from build123d import *

# Parameters (mm, degrees)
SKETCH_1_R      = 1.5
EXTRUDE_1_DEPTH = 3


with BuildPart() as part:
    # 스케치1 → 보스-돌출1 (new body)
    with BuildSketch(Plane.XY):
        Polygon((-47.224852071, 90.964497041), (191.775147929, 90.964497041), (191.775147929, -71.035502959), (-158.224852071, -71.035502959), (-158.224852071, 90.964497041), (-158.224852071, 112.964497041), (-47.224852071, 112.964497041), align=None)
        with Locations((-108.224852071, 78.964497041)):
            Circle(SKETCH_1_R, mode=Mode.SUBTRACT)
        with Locations((-68.224852071, 78.964497041)):
            Circle(SKETCH_1_R, mode=Mode.SUBTRACT)
        with Locations((101.775147929, 78.964497041)):
            Circle(SKETCH_1_R, mode=Mode.SUBTRACT)
        with Locations((141.775147929, 78.964497041)):
            Circle(SKETCH_1_R, mode=Mode.SUBTRACT)
        with Locations((141.775147929, -41.035502959)):
            Circle(SKETCH_1_R, mode=Mode.SUBTRACT)
        with Locations((41.775147929, -41.035502959)):
            Circle(SKETCH_1_R, mode=Mode.SUBTRACT)
        with Locations((-8.224852071, -41.035502959)):
            Circle(SKETCH_1_R, mode=Mode.SUBTRACT)
        with Locations((-108.224852071, -41.035502959)):
            Circle(SKETCH_1_R, mode=Mode.SUBTRACT)
        with Locations((-152.024852071, 110.064497041)):
            Circle(SKETCH_1_R, mode=Mode.SUBTRACT)
        with Locations((-50.424852071, 110.064497041)):
            Circle(SKETCH_1_R, mode=Mode.SUBTRACT)
        with Locations((-41.224852071, 86.464497041)):
            Circle(SKETCH_1_R, mode=Mode.SUBTRACT)
        with Locations((185.775147929, 86.464497041)):
            Circle(SKETCH_1_R, mode=Mode.SUBTRACT)
        with Locations((185.775147929, -64.535502959)):
            Circle(SKETCH_1_R, mode=Mode.SUBTRACT)
        with Locations((-41.224852071, -64.535502959)):
            Circle(SKETCH_1_R, mode=Mode.SUBTRACT)
        with Locations((-50.424852071, -64.535502959)):
            Circle(SKETCH_1_R, mode=Mode.SUBTRACT)
        with Locations((-152.024852071, -64.535502959)):
            Circle(SKETCH_1_R, mode=Mode.SUBTRACT)
    extrude(amount=EXTRUDE_1_DEPTH)


solid = part.part
Can you work these out from the model? Positions are in its coordinate system, mm. Coordinates: 2 decimals unless noted, no trailing zeros. Write each loop counter-clockwise with the first axis right and the second up, starting at its lowest first coordinate (ties: lowest second). Pieces come first, ordered by that corner, then holes. Notation, with made-up numbers: (48.5, 9) - (71.5, 9) arc R24 ccw to (71.5, 32) - close; hole circle Ø9 at (-28, 23.25). An arc over 180 degrees is marked (long way). Return JSON: item names as keys, results as strings. Group by question number.
Item 1: If we section it at A-A (x = 71): Write out the boundary of the cut face in (y, z).
Item 2: I'm going to push flat-ended pins straight in: pin 1 Ø4 at (x, y) = (-50.42, -64.54) entering from +Z; pin 2 Ø0.9 at (x, z) = (84, 2) entering from +Y. Where does each tip first touch, or does it pass through?
Item 3: If we section it at B-B (z = 1.05): Count the separate pieces of the cut face and the enclosed holes in it, then the cut area to 3 significant figures.
Item 4: Please list where these lines run through material, in increasing order: probe 1 along Y at (x, z) = (-49.5, 0.7); probe 2 along Y at (x, z) = (52, 0.4); probe 3 along X at (y, z) = (100.5, 2.1).
Return value:
{
 "1": {"outline": "(-71.04, 0) - (90.96, 0) - (90.96, 3) - (-71.04, 3) - close"},
 "2": {"pin 1": "stops at z = 3", "pin 2": "stops at y = 90.96"},
 "3": {"separate pieces": "1", "enclosed holes": "16", "area": "59,000 mm^2"},
 "4": {"probe 1": "y = -71.04 to -65.72, -63.35 to 108.88, 111.25 to 112.96", "probe 2": "y = -71.04 to 90.96", "probe 3": "x = -158.22 to -47.22"}
}
